from build123d import *

# Parameters (mm, degrees)
SKETCH1_W               = 673.1
SKETCH1_H               = 965.2
BOSS_EXTRUDE1_DEPTH     = 7.9375
CUT_EXTRUDE1_DEPTH      = 1
CUT_EXTRUDE1_DEPTH_BACK = 16.875
CUT_EXTRUDE2_DEPTH      = 674.1
SKETCH4_W               = 7.9375
SKETCH4_H               = 936.625
BOSS_EXTRUDE2_DEPTH     = 15.875
FILLET1_R               = 6.35
SKETCH5_R               = 1.5875
CUT_EXTRUDE3_DEPTH      = 8
SKETCH6_R               = 4.826
CUT_EXTRUDE4_DEPTH      = 16.875


with BuildPart() as part:
    # Sketch1 → Boss-Extrude1 (new body, symmetric)
    with BuildSketch(Plane.XY):
        Rectangle(SKETCH1_W, SKETCH1_H)
    extrude(amount=BOSS_EXTRUDE1_DEPTH, both=True)

    # Sketch2 → Cut-Extrude1 (cut, two sides)
    with BuildSketch(Plane.XY.offset(7.9375)) as cut_extrude1_sk:
        with BuildLine():
            Line((-230.32810678, -204.086249688), (-84.27810678, -204.086249688))
            ThreePointArc((-84.27810678, -204.086249688), (-82.03304275, -205.016185658), (-81.10310678, -207.261249688))
            Line((-81.10310678, -207.261249688), (-81.10310678, -302.511249688))
            ThreePointArc((-81.10310678, -302.511249688), (-82.03304275, -304.756313718), (-84.27810678, -305.686249688))
            Line((-84.27810678, -305.686249688), (-230.32810678, -305.686249688))
            ThreePointArc((-230.32810678, -305.686249688), (-232.57317081, -304.756313718), (-233.50310678, -302.511249688))
            Line((-233.50310678, -302.511249688), (-233.50310678, -207.261249688))
            ThreePointArc((-233.50310678, -207.261249688), (-232.57317081, -205.016185658), (-230.32810678, -204.086249688))
        make_face()
        with BuildLine():
            Line((81.10310678, -207.261249688), (81.10310678, -302.511249688))
            ThreePointArc((81.10310678, -302.511249688), (82.03304275, -304.756313718), (84.27810678, -305.686249688))
            Line((84.27810678, -305.686249688), (230.32810678, -305.686249688))
            ThreePointArc((230.32810678, -305.686249688), (232.57317081, -304.756313718), (233.50310678, -302.511249688))
            Line((233.50310678, -302.511249688), (233.50310678, -207.261249688))
            ThreePointArc((233.50310678, -207.261249688), (232.57317081, -205.016185658), (230.32810678, -204.086249688))
            Line((230.32810678, -204.086249688), (84.27810678, -204.086249688))
            ThreePointArc((84.27810678, -204.086249688), (82.03304275, -205.016185658), (81.10310678, -207.261249688))
        make_face()
    extrude(amount=CUT_EXTRUDE1_DEPTH, mode=Mode.SUBTRACT)
    extrude(cut_extrude1_sk.sketch, amount=-CUT_EXTRUDE1_DEPTH_BACK, mode=Mode.SUBTRACT)

    # Sketch3 → Cut-Extrude2 (cut, through all)
    with BuildSketch(Plane(origin=(336.55, 0, 0), x_dir=(0, 0, -1), z_dir=(1, 0, 0))):
        Polygon((-7.9375, 482.6), (7.9375, 479.800809181), (7.9375, 482.6), align=None)
    extrude(amount=-CUT_EXTRUDE2_DEPTH, mode=Mode.SUBTRACT)

    # Sketch4 → Boss-Extrude2 (add)
    with BuildSketch(Plane.XY.offset(7.9375)):
        with Locations((-340.51875, 0)):
            Rectangle(SKETCH4_W, SKETCH4_H)
        with Locations((340.51875, 0)):
            Rectangle(SKETCH4_W, SKETCH4_H)
    extrude(amount=-BOSS_EXTRUDE2_DEPTH)

    # Fillet1
    fillet1_edges = [part.edges().sort_by_distance(p)[0] for p in [
        (-336.55, -468.3125, 0),
        (-336.55, 468.3125, 0),
        (336.55, 468.3125, 0),
        (336.55, -468.3125, 0),
    ]]
    fillet(fillet1_edges, radius=FILLET1_R)

    # Sketch5 → Cut-Extrude3 (cut)
    with BuildSketch(Plane.XY.offset(7.9375)):
        with Locations((-316, -257.871720704)):
            Circle(SKETCH5_R)
        with Locations((-284, -257.871720704)):
            Circle(SKETCH5_R)
        with Locations((-300, -280.871720704)):
            Circle(SKETCH5_R)
        with Locations((-16, -257.871720704)):
            Circle(SKETCH5_R)
        with Locations((16, -257.871720704)):
            Circle(SKETCH5_R)
        with Locations((0, -280.871720704)):
            Circle(SKETCH5_R)
        with Locations((284, -257.871720704)):
            Circle(SKETCH5_R)
        with Locations((300, -280.871720704)):
            Circle(SKETCH5_R)
        with Locations((316, -257.871720704)):
            Circle(SKETCH5_R)
    extrude(amount=-CUT_EXTRUDE3_DEPTH, mode=Mode.SUBTRACT)

    # Sketch6 → Cut-Extrude4 (cut, through all)
    with BuildSketch(Plane(origin=(0, 0, -7.9375), x_dir=(-1, 0, 0), z_dir=(0, 0, -1))):
        with Locations((-234.95, 400.05)):
            Circle(SKETCH6_R)
        with Locations((-71.966666709, 400.05)):
            Circle(SKETCH6_R)
        with Locations((71.966666709, 400.05)):
            Circle(SKETCH6_R)
        with Locations((234.95, 400.05)):
            Circle(SKETCH6_R)
        with Locations((-234.95, -28.575)):
            Circle(SKETCH6_R)
        with Locations((-71.966666709, -28.575)):
            Circle(SKETCH6_R)
        with Locations((71.966666709, -28.575)):
            Circle(SKETCH6_R)
        with Locations((234.95, -28.575)):
            Circle(SKETCH6_R)
    extrude(amount=-CUT_EXTRUDE4_DEPTH, mode=Mode.SUBTRACT)


solid = part.part
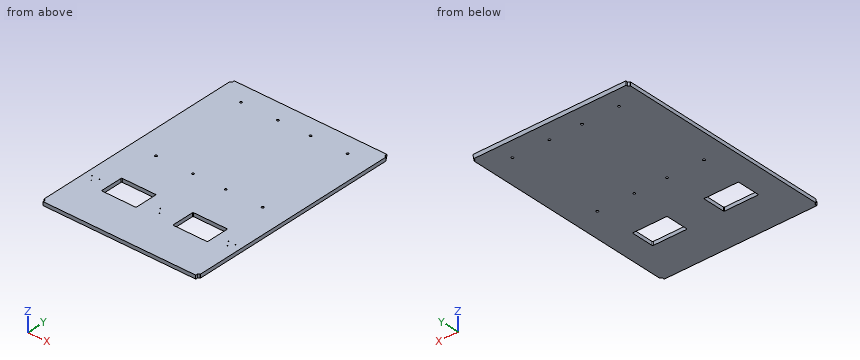
Can you work these out from the model? Positions are in its coordinate system, mm. Give positions to 0.01 mm unless a question says otherwise; leave off trailing zeros. Loops run counter-clockwise (first coordinate to the right, second up) from the corner with the lowest first, then second, coordinate; pieces in that order, holes last. Notation, with made-up numbers: (65, 19) - (101, 19) arc R23 cw to (101, 40) - close; hole circle Ø5 at (-8.5, 57.5). An arc over 180 degrees is marked (long way). Return JSON: item names as keys, results as strings.
1. I'm going to push flat-ended pins straight in: pin 1 Ø12.5 at (x, y) = (-71.97, 400.05) entering from +Z; pin 2 Ø8.5 at (y, z) = (-479, 1) entering from -X; pin 3 Ø1.6 at (x, y) = (-300.5, -280.5) entering from +Z; pin 4 Ø6 at (x, y) = (234.95, 400.05) entering from -Z. Where does each tip first touch, or does it pass through?
Output values:
{"pin 1": "stops at z = 7.94", "pin 2": "stops at x = -336.55", "pin 3": "stops at z = -0.06", "pin 4": "passes through"}
2. If I drill on line 1 (X direction, y = -279, z = 3.75); line 2 (Y direction, x = 191, z = 7.25); line 3 (Y direction, x = 86, z = -6.75), over which ranges is the centre line in solid material (lowest first)?
Output values:
{"line 1": "x = -344.49 to -233.5, -81.1 to 81.1, 233.5 to 344.49", "line 2": "y = -482.6 to -305.69, -204.09 to 482.48", "line 3": "y = -482.6 to -305.69, -204.09 to 480.01"}
3. I want a section at B-B on z = -3. Give the number of separate pieces and of enclosed holes in the cut face, and give its area (3 significant figures).
Output values:
{"separate pieces": "1", "enclosed holes": "10", "area": "632,000 mm²"}
4. I want a section at A-A on y = -222. Please give me the cut outline in (x, z).
Output values:
{"outline": "(-344.49, -7.94) - (-233.5, -7.94) - (-233.5, 7.94) - (-344.49, 7.94) - close; (-81.1, -7.94) - (81.1, -7.94) - (81.1, 7.94) - (-81.1, 7.94) - close; (233.5, -7.94) - (344.49, -7.94) - (344.49, 7.94) - (233.5, 7.94) - close"}
